```python
from build123d import *

# Parameters (mm, degrees)
CROQUIS1_R              = 2
SALIENTE_EXTRUIR1_DEPTH = 5


with BuildPart() as part:
    # Croquis1 → Saliente-Extruir1 (new body)
    with BuildSketch(Plane.XY):
        Polygon((0, 3), (3, 0), (0, -3), (-3, 0), align=None)
        Circle(CROQUIS1_R, mode=Mode.SUBTRACT)
    extrude(amount=SALIENTE_EXTRUIR1_DEPTH)


solid = part.part
```
Input: part model. Units: mm. Frame: model coordinates. Coordinates: 2 decimals unless noted, no trailing zeros. Loops run counter-clockwise (first coordinate to the right, second up) from the corner with the lowest first, then second, coordinate; pieces in that order, holes last. Notation, with made-up numbers: (42.25, 75.5) - (64.25, 75.5) arc R30 ccw to (64.25, 109.5) - close; hole circle Ø5 at (47.5, 83). An arc over 180 degrees is marked (long way). Answer in a Markdown table with one row per item.
(1) Material intervals for L1, parallel to X at y = -0.95, z = 2.7; L2, parallel to Y at x = 0.9, z = 1.3; L3, parallel to X at y = -0.6, z = 3.75, sorted ascending. Write a range as from..to.
Model answer:
| item | result |
|---|---|
| L1 | x = -2.05..-1.76, 1.76..2.05 |
| L2 | y = -2.1..-1.79, 1.79..2.1 |
| L3 | x = -2.4..-1.91, 1.91..2.4 |
(2) Cut plane C-C on x = -0.35. Output: boundary loops of the cut face in (y, z), plus the area to 3 significant figures.
Model answer:
| item | result |
|---|---|
| outline | (-2.65, 0) - (-1.97, 0) - (-1.97, 5) - (-2.65, 5) - close; (1.97, 0) - (2.65, 0) - (2.65, 5) - (1.97, 5) - close |
| area | 6.81 mm² |
(3) Mould query, pull axis Y, two halves, no side actions, for faces 1 (the face through (1, 2, 2)), 2 (the face through (0, -2, 2)), 3 (the face through (-1, -2, 2)). Classes: pulls with the +Y half, pulls with the -Y half, needs draft (parallel to the pull), parting line crosses it, or undercut.
Model answer:
| item | result |
|---|---|
| face 1 | pulls with the +Y half |
| face 2 | undercut |
| face 3 | pulls with the -Y half |
(4) Cut plane A-A on z = 1.3. Output: boundary loops of the cut face in (x, y).
Model answer:
| item | result |
|---|---|
| outline | (-3, 0) - (0, -3) - (3, 0) - (0, 3) - close; hole circle Ø4 at (0, 0) |
(5) Cut plane B-B on y = -1.8. Output: boundary loops of the cut face in (x, z), plus the area to 3 significant figures.
Model answer:
| item | result |
|---|---|
| outline | (-1.2, 0) - (-0.87, 0) - (-0.87, 5) - (-1.2, 5) - close; (0.87, 0) - (1.2, 0) - (1.2, 5) - (0.87, 5) - close |
| area | 3.28 mm² |
